Geometry: see drawing. Coordinates: mm, zero at the bounding-box minimum. A direction names the side the tool comes from. Give positions to 0.01 mm unless a question says otherwise; leave off trailing zeros. Write each loop counter-clockwise with the first axis right and the second up, starting at its lowest first coordinate (ties: lowest second). Pieces come first, ordered by that corner, then holes.
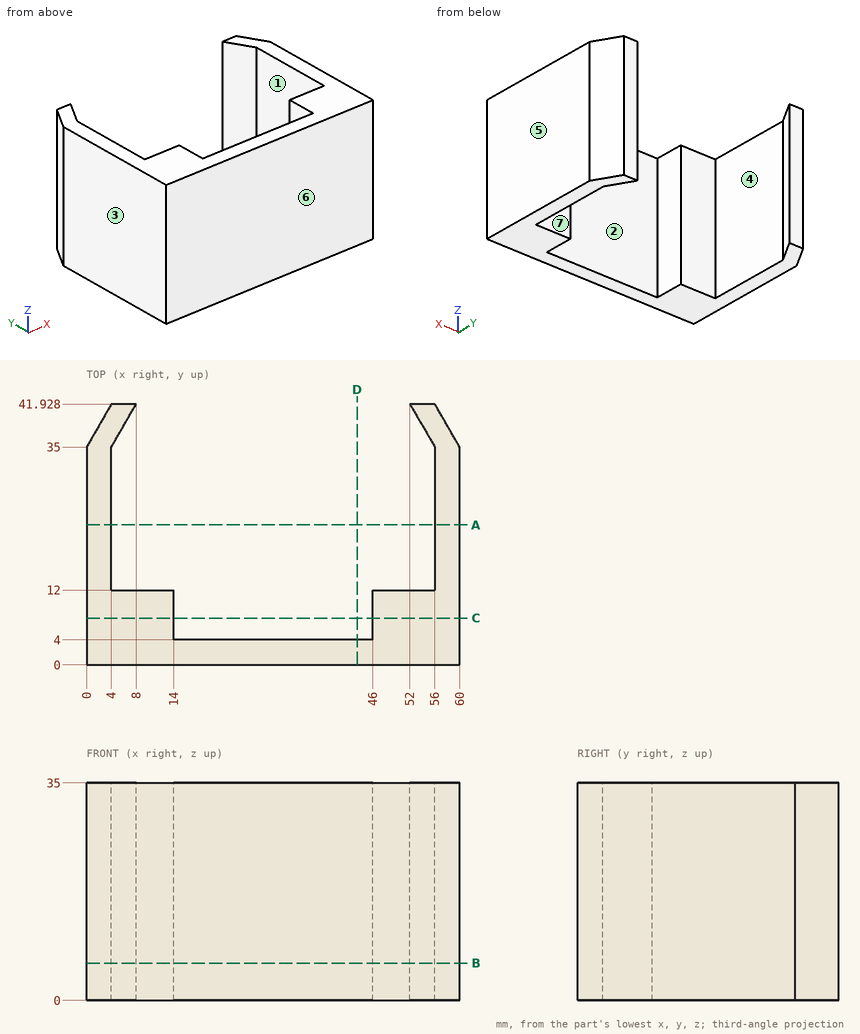
Q1. Pin query (flat end, axial travel): pin 1 (1 mm diameter, centred on x = 32.5, y = 6, fed in from +Z). Return the tip coordinate at first contact, or that it passes through.
Q2. Access query for the marked faces 1, 2 and 3. Directions: +Z, -Z, +X, -X, +Y, -Y. A direction counts if a zero-diameter tool reaches every point of the face in a straight line with its end or side. Return the directions, or none.
Q3. Mould query, pull axis X, two halves, no side actions, for the marked faces 4, 5, 6 and 7. Classes: +X half, -X half, draft (parallel to the pull), parting line (faces both ways), or undercut.
Q4. Section D-D, the plane x = 43.5. Return the cut outline in (y, z).
Q5. Section A-A, the plane y = 22.5. Return the cut outline in (x, z), then the cut area to 3 significant figures.
Q6. Material intervals for line 1 along X through (y, z) = (33, 24); line 2 along X through (y, z) = (5, 24); line 3 along Y through (x, z) = (13, 4), sorted ascending.
Q7. Section B-B, the plane z = 6. Return the cut outline in (x, y).
Q8. Section C-C, the plane y = 7.5. Return the cut outline in (x, z).
Solutions:
1. pin 1: passes through
2. face 1: +Z, -Z
2. face 2: +Z, -Z, +Y
2. face 3: +Z, -Z, -X, +Y, -Y
3. face 4: undercut
3. face 5: +X half
3. face 6: draft
3. face 7: undercut
4. outline: (0, 0) - (4, 0) - (4, 35) - (0, 35) - close
5. outline: (0, 0) - (4, 0) - (4, 35) - (0, 35) - close; (56, 0) - (60, 0) - (60, 35) - (56, 35) - close
5. area: 280 mm2
6. line 1: x = 0 to 4, 56 to 60
6. line 2: x = 0 to 14, 46 to 60
6. line 3: y = 0 to 12
7. outline: (0, 0) - (60, 0) - (60, 35) - (56, 41.93) - (52, 41.93) - (56, 35) - (56, 12) - (46, 12) - (46, 4) - (14, 4) - (14, 12) - (4, 12) - (4, 35) - (8, 41.93) - (4, 41.93) - (0, 35) - close
8. outline: (0, 0) - (14, 0) - (14, 35) - (0, 35) - close; (46, 0) - (60, 0) - (60, 35) - (46, 35) - close
